Autodesk Inventor part; units mm, degrees
ref_plane "YZ Plane" through (0, 0, 0) normal (1, 0, 0) x (0, 1, 0)
ref_plane "XZ Plane" through (0, 0, 0) normal (0, 1, 0) x (-1, 0, 0)
ref_plane "XY Plane" through (0, 0, 0) normal (0, 0, 1) x (1, 0, 0)
sketch "Sketch3" plane through (0, 0, 0) normal (0, 1, 0) x (-1, 0, 0)
  arc A0 (0, 10) -> (-10, 0) centre (0, 0) ccw
  arc A1 (0, 12) -> (-12, 0) centre (0, 0) ccw
  line L0 (0, 10) -> (2, 10)
  line L1 (2, 10) -> (2, 19)
  line L2 (2, 19) -> (0, 19)
  line L3 (0, 19) -> (0, 10)
  line L4 (-10, 0) -> (-19, 0)
  line L5 (-19, 0) -> (-19, -2)
  line L6 (-19, -2) -> (-10, -2)
  line L7 (-10, -2) -> (-10, 0)
  line L8 (0, 12) -> (0, 10)
  line L9 (-10, 0) -> (-12, 0)
  dimension "d10" = 10
  dimension "d11" = 12
  dimension "d12" = 2
  dimension "d13" = 9
  dimension "d14" = 9
  dimension "d15" = 2
extrude "Extrusion2" add sketch "Sketch3" along normal blind 7
sketch "Sketch4" plane through (0, 0, 19) normal (1, 0, 0) x (0, 0, -1)
  line L0 (0, 0) -> (0, 7)
  line L1 (0, 3.5) -> (7, 3.5) construction
  line L2 (7, 0) -> (7, 7)
  line L3 (7, 0) -> (7, 7) construction
  line L4 (0, 7) -> (7, 7) construction
  line L5 (0, 0) -> (0, 7) construction
  line L6 (0, 0) -> (7, 0) construction
  line L7 (9, 7) -> (0, 7) construction
  line L8 (3.5, 7) -> (3.5, 3.5) construction
  circle A0 centre (3.5, 3.5) radius 1.15
  point P0 (19, 0)
  dimension "d18" = 2.3
extrude "Extrusion3" cut sketch "Sketch4" against normal blind 2
chamfer "Chamfer1" distance 1.5 angle 45 1 edges at (0, 3.5, 16.65)
sketch "Sketch6" plane through (12, 0, 0) normal (0, 0, 1) x (1, 0, 0)
  line L0 (7, 0) -> (7, 7)
  line L1 (7, 3.5) -> (0.0163, 3.5) construction
  line L2 (0, 7) -> (7, 7)
  line L3 (3.5, 7) -> (3.5082, 3.5) construction
  circle A0 centre (3.5082, 3.5) radius 1.15
  point P0 (-12, 0)
  dimension "d24" = 2.3
extrude "Extrusion4" cut sketch "Sketch6" against normal blind 2
chamfer "Chamfer2" distance 1.5 angle 45 1 edges at (14.3582, 3.5, 0)
properties part number "wiresHolder"
Source: CAD feature listing. Evaluate the final solid. Frame: model axes, mm. A direction names the side the tool comes from. Coordinates: 2 decimals unless noted, no trailing zeros. Loops run counter-clockwise (first coordinate to the right, second up) from the corner with the lowest first, then second, coordinate; pieces in that order, holes last. Notation, with made-up numbers: (26.25, -4) -> (56.25, -4) arc R9 cw to (56.25, 12) -> close; hole circle Ø7 at (56.5, 58). An arc over 180 degrees is marked (long way). Answer in a Markdown table with one row per item. Add a question column.
Q1. Contact query for flat-ended pins moving along their axis: pin 1 Ø2 at (x, y) = (3, 3) entering from -Z; pin 2 Ø2 at (y, z) = (2, 14.5) entering from +X; pin 3 Ø0.6 at (y, z) = (3, -1) entering from -X; pin 4 Ø1.8 at (x, y) = (15.51, 3.5) entering from -Z. Output: stop coordinate, or through.
Q2. Pull-direction query (Z, two-part tool) for faces 1 (the face through (8.58, 3.45, 8.39)), 2 (the face through (8, 0, 7)), 3 (the face through (-1.75, 3.55, 16.65)); classes: pulls with the +Z half, pulls with the -Z half, needs draft (parallel to the pull), parting line crosses it, or undercut.
Q3. Ray query, line 1 along Y through (x, z) = (-1.75, 15.5); line 2 along Z through (x, y) = (13.75, 6); line 3 along X through (y, z) = (4.5, 0.25). Return the intervals inside material, ascending.
Q4. Reachability of faces 4 (the face through (14.596, 2.8, -1.746)), 5 (the face through (10, 3, -1)), 6 (the face through (18, 5, 0)) from +Z, -Z, +X, -X, +Y, -Y: full face, straight path, thin tool, end or side. Return the list, or none.
Q5. Section D-D on y = 0.5. Return the cut outline in (x, z).
Q6. Section B-B on z = 15.5. Return the cut outline in (x, y).
Q7. Section C-C on x = -0.5. Return the cut outline in (y, z).
Q8. Section A-A on y = 3.5. Return the cut outline in (x, z).
Computed values:
| question | item | result |
|---|---|---|
| 1 | pin 1 | stops at z = 9.17 |
| 1 | pin 2 | stops at x = 0 |
| 1 | pin 3 | stops at x = 10 |
| 1 | pin 4 | passes through |
| 2 | face 1 | pulls with the +Z half |
| 2 | face 2 | needs draft |
| 2 | face 3 | undercut |
| 3 | line 1 | y = 0 to 2.35, 4.65 to 7 |
| 3 | line 2 | z = -2 to 0 |
| 3 | line 3 | x = 10 to 12 |
| 4 | face 4 | +Z, -Z |
| 4 | face 5 | -Z, -X, +Y, -Y |
| 4 | face 6 | +Z, +X, +Y, -Y |
| 5 | outline | (-2, 10) -> (0, 10) arc R10 cw to (10, 0) -> (10, -2) -> (19, -2) -> (19, 0) -> (12, 0) arc R12 ccw to (0, 12) -> (0, 19) -> (-2, 19) -> close |
| 6 | outline | (-2, 0) -> (0, 0) -> (0, 0.85) -> (-1.5, 2.35) -> (-2, 2.35) -> close; (-2, 4.65) -> (-1.5, 4.65) -> (0, 6.15) -> (0, 7) -> (-2, 7) -> close |
| 7 | outline | (0, 10) -> (7, 10) -> (7, 19) -> (0, 19) -> close; hole circle Ø4.3 at (3.5, 15.5) |
| 8 | outline | (-2, 10) -> (0, 10) arc R10 cw to (10, 0) -> (10, -2) -> (14.36, -2) -> (14.36, -1.5) -> (12.86, 0) -> (12, 0) arc R12 ccw to (0, 12) -> (0, 12.85) -> (-1.5, 14.35) -> (-2, 14.35) -> close; (-2, 16.65) -> (-1.5, 16.65) -> (0, 18.15) -> (0, 19) -> (-2, 19) -> close; (16.66, -2) -> (19, -2) -> (19, 0) -> (18.16, 0) -> (16.66, -1.5) -> close |
